Can you work these out from the drawing? Everything is in mm from the part's minimum corner. A direction names the side the tool comes from. Round coordinates to 2 decimals unless told otherwise and drop trailing zeros. Write each loop counter-clockwise with the first axis right and the second up, starting at its lowest first coordinate (ties: lowest second). Pieces come first, ordered by that corner, then holes.
Q1. If we section it at C-C (y = 6.35): Please give me the cut outline in (x, z) (1 decimal).
Q2. Please list where these lines run through material, in increasing order: line 1 along X through (y, z) = (6.25, 48) (1 decimal); line 2 along Y through (x, z) = (38, 30.5) (1 decimal); line 3 along Z through (x, y) = (21, 1) (1 decimal).
Q3. If we section it at D-D (z = 6.35): Give the number of separate pieces and of enclosed holes in the cut face, plus the area to 3 significant figures.
Q4. If we section it at B-B (z = 17.5): Please give me the cut outline in (x, y) (1 decimal).
Q5. I'm going to push flat-ended pins straight in: pin 1 Ø5 at (x, z) = (4.76, 6.35) entering from -Y; pin 2 Ø3 at (x, y) = (15.875, 6.35) entering from -Z (1 decimal). Where does each tip first touch, or does it pass through?
Q6. For the marked faces 1 and 2, which set-ups out of +Z, -Z, +X, -X, +Y, -Y let a thin tool reach every point of the face, with its end or its side?
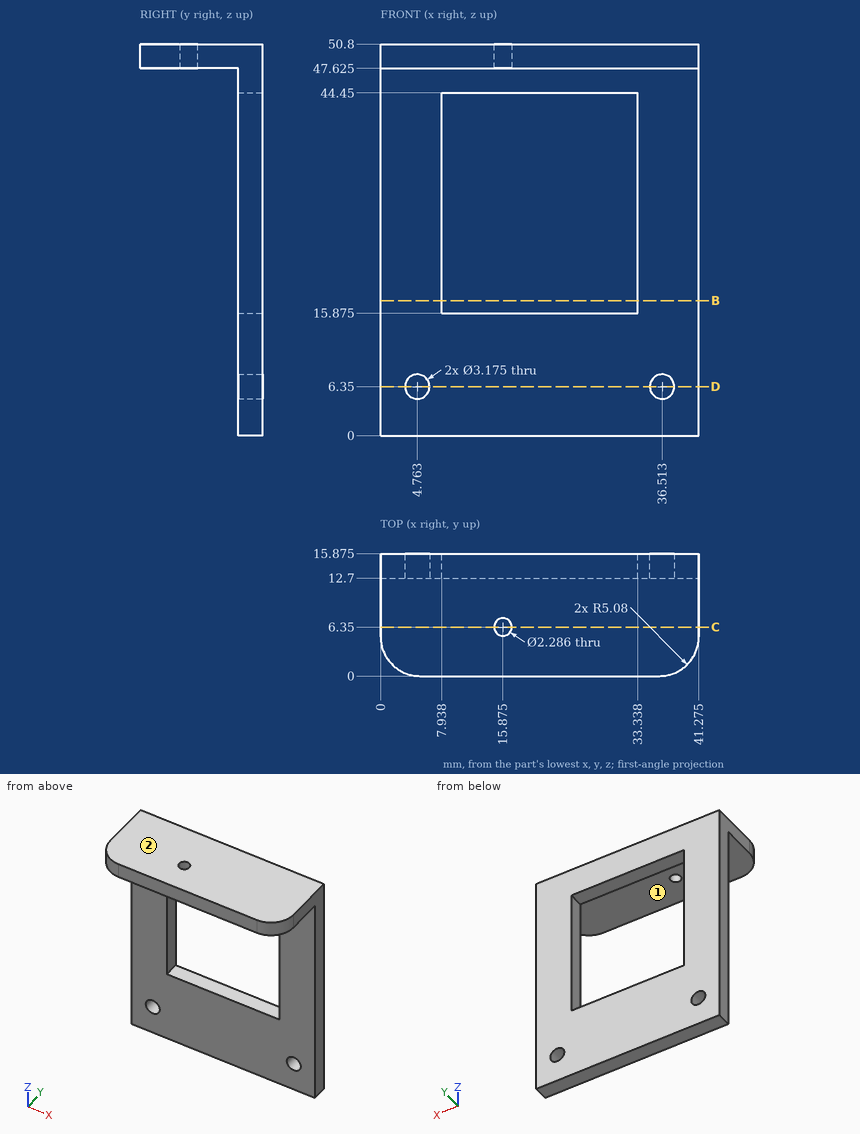
A:
1. outline: (0, 47.6) - (14.7, 47.6) - (14.7, 50.8) - (0, 50.8) - close; (17, 47.6) - (41.3, 47.6) - (41.3, 50.8) - (17, 50.8) - close
2. line 1: x = 0 to 14.7, 17 to 41.3
2. line 2: y = 12.7 to 15.9
2. line 3: z = 47.6 to 50.8
3. separate pieces: 3
3. enclosed holes: 0
3. area: 111 mm2
4. outline: (0, 12.7) - (7.9, 12.7) - (7.9, 15.9) - (0, 15.9) - close; (33.3, 12.7) - (41.3, 12.7) - (41.3, 15.9) - (33.3, 15.9) - close
5. pin 1: stops at y = 12.7
5. pin 2: stops at z = 47.6
6. face 1: -Z, +X, -X, -Y
6. face 2: +Z, +X, -X, +Y, -Y
